Check sheet for the modelled part. Datum: model origin and axes. Units: mm. A direction names the side the tool comes from. Give positions to 0.01 mm unless a question says otherwise; leave off trailing zeros. Order: outer loops, then holes, each group sorted by start corner. A loop starts at its lowest first (then second) coordinate and runs counter-clockwise, first axis right, second up.
```python
from build123d import *

# Parameters (mm, degrees)
SKETCH1_R           = 93.726
BOSS_EXTRUDE1_DEPTH = 4.826
SKETCH4_R           = 85.725
SKETCH4_R_2         = 79.375
BOSS_EXTRUDE2_DEPTH = 12.7


with BuildPart() as part:
    # Sketch1 → Boss-Extrude1 (new, symmetric)
    with BuildSketch(Plane(origin=(0, 0, 0), x_dir=(1, 0, 0), z_dir=(0, 1, 0))):
        with Locations(Location((0, 0, 0), (0, 0, 270))):
            Circle(SKETCH1_R)
    extrude(amount=BOSS_EXTRUDE1_DEPTH, both=True)

    # Sketch4 → Boss-Extrude2 (add)
    with BuildSketch(Plane(origin=(0, 4.826, 0), x_dir=(1, 0, 0), z_dir=(0, 1, 0))):
        with Locations(Location((0, 0, 0), (0, 0, 270))):
            Circle(SKETCH4_R)
        with Locations(Location((0, 0, 0), (0, 0, 270))):
            Circle(SKETCH4_R_2, mode=Mode.SUBTRACT)
    boss_extrude2 = extrude(amount=BOSS_EXTRUDE2_DEPTH)

    # Mirror2: Boss-Extrude2 across plane
    add(boss_extrude2.mirror(Plane.ZX))


solid = part.part
```
(1) Material ranges on L1, parallel to X at y = 12, z = 0 (3 decimals); L2, parallel to Y at x = 62.5, z = -8.5; L3, parallel to Z at x = -40, y = -11, recorded low to high.
Response values:
L1: x = -85.725 to -79.375, 79.375 to 85.725
L2: y = -4.83 to 4.83
L3: z = -75.82 to -68.56, 68.56 to 75.82
(2) Cross-section at B-B on x = 0. Enter the section's corners in (y, z) (3 decimals).
Response values:
outline: (-17.526, -85.725) - (-4.826, -85.725) - (-4.826, -93.726) - (4.826, -93.726) - (4.826, -85.725) - (17.526, -85.725) - (17.526, -79.375) - (4.826, -79.375) - (4.826, 79.375) - (17.526, 79.375) - (17.526, 85.725) - (4.826, 85.725) - (4.826, 93.726) - (-4.826, 93.726) - (-4.826, 85.725) - (-17.526, 85.725) - (-17.526, 79.375) - (-4.826, 79.375) - (-4.826, -79.375) - (-17.526, -79.375) - close
(3) Cross-section at C-C on y = -12.5. Enter the section's corners in (x, z) (3 decimals), then the cut area to 3 significant figures.
Response values:
outline: circle Ø171.45 at (0, 0); hole circle Ø158.75 at (0, 0)
area: 3,290 mm2
(4) Set-up check for faces 1 (the face through (-76, 17.526, 25)), 2 (the face through (-41, -4.826, 76)), 3 (the face through (23.84, 11.09, 75.71)): record each of +Z, -Z, +X, -X, +Y, -Y from which the full face is reachable in a straight line by a thin tool's end or side.
Response values:
face 1: +Z, -Z, +X, -X, +Y
face 2: -Y
face 3: +Y
(5) Cross-section at A-A on z = 0. Enter the section's corners in (x, y) (3 decimals).
Response values:
outline: (-93.726, -4.826) - (-85.725, -4.826) - (-85.725, -17.526) - (-79.375, -17.526) - (-79.375, -4.826) - (79.375, -4.826) - (79.375, -17.526) - (85.725, -17.526) - (85.725, -4.826) - (93.726, -4.826) - (93.726, 4.826) - (85.725, 4.826) - (85.725, 17.526) - (79.375, 17.526) - (79.375, 4.826) - (-79.375, 4.826) - (-79.375, 17.526) - (-85.725, 17.526) - (-85.725, 4.826) - (-93.726, 4.826) - close
(6) Release check for a two-part mould opening along Z. For faces 4 (the face through (23.84, -11.09, 75.71)), 5 (the face through (-52.2, -11.1, -68)), 6 (the face through (-41, 4.826, 76)) record: released by +Z, released by -Z, zero draft, split by the parting line, or undercut.
Response values:
face 4: undercut
face 5: split by the parting line
face 6: zero draft
(7) Gauge pin test, flat ends, axial feed: pin 1 Ø10 at (x, z) = (64.5, -61) entering from -Y; pin 2 Ø5 at (y, z) = (-5.5, 40.5) entering from -X; pin 3 Ø3 at (x, z) = (-61.5, -34) entering from -Y; pin 4 Ø1 at (x, y) = (-47.5, 8) entering from +Z. Record the tip position at first contact, or that the pin passes through.
Response values:
pin 1: stops at y = -17.53
pin 2: stops at x = -85.64
pin 3: stops at y = -4.83
pin 4: stops at z = 71.69
